from build123d import *

# Parameters (mm, degrees)
SKETCH1_R           = 39.37
BOSS_EXTRUDE1_DEPTH = 101.6
SKETCH2_R           = 31.75
CUT_EXTRUDE1_DEPTH  = 116.855745649
CUT_EXTRUDE2_START  = -33.02
SKETCH3_R           = 39.37
SKETCH3_R_2         = 34.925
CUT_EXTRUDE2_DEPTH  = 33.02
CUT_EXTRUDE3_DEPTH  = 12.7
SKETCH9_R           = 39.558823483
CUT_EXTRUDE5_DEPTH  = 111.768173967
SKETCH10_R          = 3.268271246
BOSS_EXTRUDE2_DEPTH = 10.16
CUT_EXTRUDE6_DEPTH  = 25.4
CIRPATTERN1_COUNT   = 4
CHAMFER1_SIZE       = 10


with BuildPart() as part:
    # Sketch1 → Boss-Extrude1 (new body)
    with BuildSketch(Plane(origin=(0, 0, 0), x_dir=(1, 0, 0), z_dir=(0, 1, 0))):
        with Locations(Location((0, 0, 0), (0, 0, 270))):
            Circle(SKETCH1_R)
    extrude(amount=BOSS_EXTRUDE1_DEPTH)

    # Sketch2 → Cut-Extrude1 (cut, through all)
    with BuildSketch(Plane(origin=(0, 101.6, 0), x_dir=(1, 0, 0), z_dir=(0, 1, 0))):
        with Locations(Location((0, 0, 0), (0, 0, 270))):
            Circle(SKETCH2_R)
    extrude(amount=-CUT_EXTRUDE1_DEPTH, mode=Mode.SUBTRACT)

    # Sketch3 → Cut-Extrude2 (cut)
    with BuildSketch(Plane(origin=(0, 101.6, 0), x_dir=(1, 0, 0), z_dir=(0, 1, 0)).offset(CUT_EXTRUDE2_START)):
        with Locations(Location((0, 0, 0), (0, 0, 270))):
            Circle(SKETCH3_R)
        with Locations(Location((0, 0, 0), (0, 0, 270))):
            Circle(SKETCH3_R_2, mode=Mode.SUBTRACT)
    extrude(amount=CUT_EXTRUDE2_DEPTH, mode=Mode.SUBTRACT)

    # Sketch5 → Cut-Extrude3 (cut)
    with BuildSketch(Plane.XZ):
        with BuildLine():
            Line((-7.112, -34.912297917), (-7.112, -38.722297917))
            ThreePointArc((-7.112, -38.722297917), (0, -39.380800166), (7.112, -38.722297917))
            Line((7.112, -38.722297917), (7.112, -34.912297917))
            ThreePointArc((7.112, -34.912297917), (0, -35.642563047), (-7.112, -34.912297917))
        make_face()
    cut_extrude3 = extrude(amount=-CUT_EXTRUDE3_DEPTH, mode=Mode.SUBTRACT)

    # Sketch9 → Cut-Extrude5 (cut, through all)
    with BuildSketch(Plane(origin=(0, 5.842, 0), x_dir=(-1, 0, 0), z_dir=(0, -1, 0))):
        Circle(SKETCH9_R)
    extrude(amount=CUT_EXTRUDE5_DEPTH, mode=Mode.SUBTRACT)

    # Sketch10 → Boss-Extrude2 (add)
    with BuildSketch(Plane.XZ.offset(-5.842)):
        with Locations(Location((-22.318582537, -27.07979346, 0), (0, 0, 270))):
            Circle(SKETCH10_R)
    extrude(amount=BOSS_EXTRUDE2_DEPTH)

    # Sketch23 → Cut-Extrude6 (cut)
    with BuildSketch(Plane.XZ.offset(-12.7)):
        with BuildLine():
            Line((0, -39.37), (0, -35.629329068))
            ThreePointArc((0, -35.629329068), (3.574027059, -35.449618058), (7.112, -34.912297917))
            Line((7.112, -34.912297917), (7.112, -38.722297917))
            ThreePointArc((7.112, -38.722297917), (3.570716384, -39.20774011), (0, -39.37))
        make_face()
    cut_extrude6 = extrude(amount=-CUT_EXTRUDE6_DEPTH, mode=Mode.SUBTRACT)

    # CirPattern1: Cut-Extrude3, Cut-Extrude6 ×4 about axis
    cirpattern1_axis = Axis((0, 0, 0), (0, 1, 0))
    add([cut_extrude3.rotate(cirpattern1_axis, i * 360 / CIRPATTERN1_COUNT) for i in range(1, CIRPATTERN1_COUNT)], mode=Mode.SUBTRACT)
    add([cut_extrude6.rotate(cirpattern1_axis, i * 360 / CIRPATTERN1_COUNT) for i in range(1, CIRPATTERN1_COUNT)], mode=Mode.SUBTRACT)

    # Chamfer1
    # the kernel refuses this chamfer: 10 mm, written as the material it takes off along each edge
    with BuildSketch(Plane(origin=(0, 68.58, 0), x_dir=(0, 0, 1), z_dir=(-1, 0, 0))) as chamfer1_piece_1_section:
        Polygon((39.37, -CHAMFER1_SIZE), (39.37 - CHAMFER1_SIZE, 0), (39.37, 0), align=None)
    chamfer1_piece_1 = revolve(axis=Axis((0, 68.58, 0), (0, 1, 0)), mode=Mode.PRIVATE)
    chamfer1_piece_1 = chamfer1_piece_1 - Plane(origin=(0, 60.807735234, 0), x_dir=(0, 0, 1), z_dir=(0, -1, 0)) * Cylinder(34.925, 158, mode=Mode.PRIVATE)
    add(chamfer1_piece_1, mode=Mode.SUBTRACT)


solid = part.part
Can you work these out from the model? Positions are in its coordinate system, mm. A direction names the side the tool comes from. Give positions to 0.01 mm unless a question says otherwise; leave off trailing zeros. Loops run counter-clockwise (first coordinate to the right, second up) from the corner with the lowest first, then second, coordinate; pieces in that order, holes last. Notation, with made-up numbers: (-28.75, 78) - (-15.75, 78) arc R22 ccw to (-15.75, 89) - close; hole circle Ø2 at (43.25, -20). An arc over 180 degrees is marked (long way). Return JSON: item names as keys, results as strings.
1. If I drill on line 1 (X direction, y = 44, z = 0); line 2 (X direction, y = 74, z = 0) (3 decimals); line 3 (Z direction, x = 0.5, y = 15), over which ranges is the centre line in solid material (lowest first)?
Output values:
{"line 1": "x = -39.37 to -31.75, 31.75 to 39.37", "line 2": "x = -34.925 to -31.75, 31.75 to 34.925", "line 3": "z = -35.63 to -31.75, 31.75 to 39.37"}
2. We'd pull the mould along Z, two halves only. Please class faces 5 (the face through (7.112, 9, 37)), 6 (the face through (-34.305, 62.809, -7.618)), 7 (the face through (37, 38.1, 4)): +Z half, -Z half, draft (parallel to the pull), parting line (faces both ways), or undercut.
Output values:
{"face 5": "draft", "face 6": "parting line", "face 7": "undercut"}
3. I'm going to push flat-ended pins straight in: pin 1 Ø2 at (x, z) = (-3, -37.5) entering from -Y; pin 2 Ø1.3 at (x, z) = (-38, -4.5) entering from -Y; pin 3 Ø12 at (y, z) = (58, 26.5) entering from -X. Where does each tip first touch, or does it pass through?
Output values:
{"pin 1": "stops at y = 12.7", "pin 2": "stops at y = 38.1", "pin 3": "stops at x = -33.61"}
4. For faces 1 (the face through (7.112, 22, -37)), 2 (the face through (4, 12.7, 37)), 3 (the face through (-37, 9, 7.112)), 4 (the face through (37, 12.7, -4)), which set-ups out of +Z, -Z, +X, -X, +Y, -Y let a thin tool reach every point of the face, with its end or its side?
Output values:
{"face 1": "-Z, -Y", "face 2": "+Z, -Y", "face 3": "-X, -Y", "face 4": "+X, -Y"}
5. I want a section at A-A on y = 67.5. Please give me the cut outline in (x, z) (3 decimals).
Output values:
{"outline": "circle Ø69.85 at (0, 0); hole circle Ø63.5 at (0, 0)"}
